Job drawing, mm, ordinate dimensions from the low corner. One solid piece. Round coordinates to 2 decimals unless told otherwise and drop trailing zeros. Loops run counter-clockwise (first coordinate to the right, second up) from the corner with the lowest first, then second, coordinate; pieces in that order, holes last.
1) Band-saw the part on B-B, the plane y = 6.5. Write the cut outline in (x, z), then the cut area to 3 significant figures.
2) Drop flat-ended pins along their axis: P1, Ø3, axis at y = 5.5, z = 254, coming from the -X side; P2, Ø1.2, axis at x = 185.5, z = 67.5, coming from the -Y side; P3, Ø5, axis at x = 222, z = 202, coming from the -Y side; P4, Ø5, axis at x = 312, y = 6.5, coming from the +Z side. Give the stop position or say it passes through.
3) Band-saw the part on D-D, the plane x = 287.5. Write the cut outline in (y, z), then the cut area to 3 significant figures.
4) Probe line 1 (Z direction, x = 180, y = 5.25); line 2 (Z direction, x = 307, y = 0.75); line 3 (X direction, y = 3, z = 293.5). List the from-to ranges inside material, lowest first.
5) Band-saw the part on A-A, the plane x = 180. Write the cut outline in (y, z), then the cut area to 3 significant figures.
6) Band-saw the part on C-C, the plane z = 90. Write the cut outline in (x, y), then the cut area to 3 significant figures.
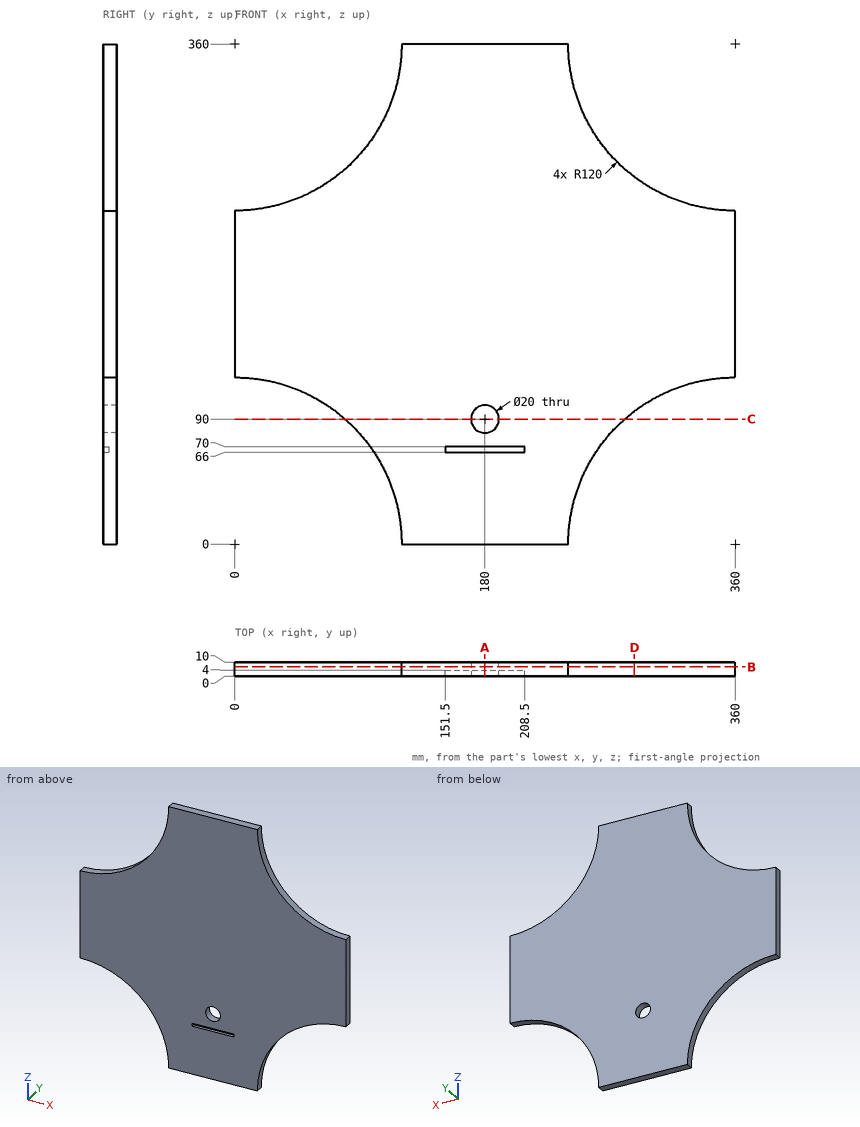
Reported:
1. outline: (0, 120) arc R120 cw to (120, 0) - (240, 0) arc R120 cw to (360, 120) - (360, 240) arc R120 cw to (240, 360) - (120, 360) arc R120 cw to (0, 240) - close; hole circle Ø20 at (180, 90)
1. area: 84,000 mm2
2. P1: stops at x = 53.33
2. P2: stops at y = 4
2. P3: stops at y = 0
2. P4: stops at z = 251.14
3. outline: (0, 95.62) - (10, 95.62) - (10, 264.38) - (0, 264.38) - close
3. area: 1,690 mm2
4. line 1: z = 0 to 80, 100 to 360
4. line 2: z = 107.66 to 252.34
4. line 3: x = 99.89 to 260.11
5. outline: (0, 0) - (10, 0) - (10, 80) - (0, 80) - (0, 70) - (4, 70) - (4, 66) - (0, 66) - close; (0, 100) - (10, 100) - (10, 360) - (0, 360) - close
5. area: 3,380 mm2
6. outline: (79.37, 0) - (170, 0) - (170, 10) - (79.37, 10) - close; (190, 0) - (280.63, 0) - (280.63, 10) - (190, 10) - close
6. area: 1,810 mm2
